Could you check a few things on this model? Use its own coordinates, in mm. Face numbers are marked on the shaded views. A direction names the side the tool comes from. Round coordinates to 2 decimals unless told otherwise and drop trailing zeros. Loops run counter-clockwise (first coordinate to the right, second up) from the corner with the lowest first, then second, coordinate; pieces in that order, holes last. Notation, with made-up numbers: (37, -21.75) -> (71, -21.75) arc R28 ccw to (71, -1.75) -> close; hole circle Ø2 at (89.25, 62.25). An arc over 180 degrees is marked (long way). Write each question's results on one line, items separated by ' | '.
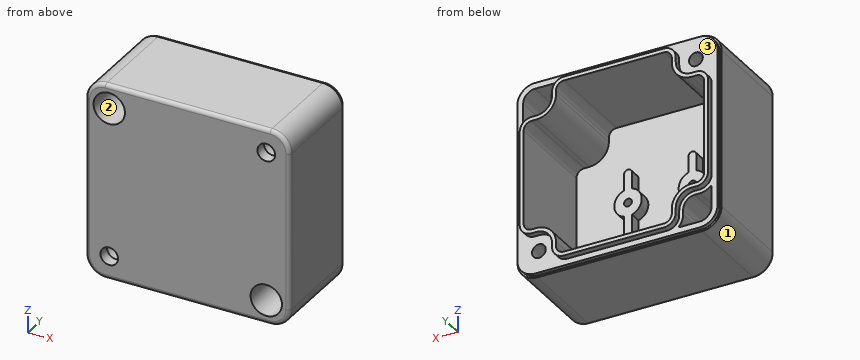
from build123d import *

# Parameters (mm, degrees)
EXTRUDE_1_DEPTH       = 25
CUT_EXTRUDE_START     = 2.5
CUT_EXTRUDE_1_DEPTH   = 22.5
CUT_EXTRUDE_START_2   = 3
CUT_EXTRUDE_3_DEPTH   = 22
EXTRUDE_START         = 25
EXTRUDE_1_2_DEPTH     = 1.6
CUT_EXTRUDE_START_3   = 25
CUT_EXTRUDE_1_2_DEPTH = 1
FILLET_1_R            = 0.2
SKETCH_9_R            = 2.25
CUT_EXTRUDE_4_DEPTH   = 4
SKETCH_10_R           = 4
CUT_EXTRUDE_5_DEPTH   = 17
FILLET_2_R            = 1
SKETCH_11_R           = 1.75
CUT_EXTRUDE_6_DEPTH   = 25
EXTRUDE_2_DEPTH       = 5.5
SKETCH_13_R           = 3.5
EXTRUDE_3_DEPTH       = 5.5
SKETCH_14_R           = 1
CUT_EXTRUDE_7_DEPTH   = 4.5


with BuildPart() as part:
    # Эскиз1 → Extrude 1 (new body)
    with BuildSketch(Plane(origin=(0, 0, 0), x_dir=(1, 0, 0), z_dir=(0, 1, 0))):
        with BuildLine():
            Line((-21, 25), (21, 25))
            ThreePointArc((21, 25), (24.535533906, 23.535533906), (26, 20))
            Line((26, 20), (26, -20))
            ThreePointArc((26, -20), (24.535533906, -23.535533906), (21, -25))
            Line((21, -25), (-21, -25))
            ThreePointArc((-21, -25), (-24.535533906, -23.535533906), (-26, -20))
            Line((-26, -20), (-26, 20))
            ThreePointArc((-26, 20), (-24.535533906, 23.535533906), (-21, 25))
        make_face()
    extrude(amount=EXTRUDE_1_DEPTH)

    # Эскиз2 → Cut-Extrude 1 (cut)
    with BuildSketch(Plane(origin=(0, 0, 0), x_dir=(1, 0, 0), z_dir=(0, 1, 0)).offset(CUT_EXTRUDE_START)):
        with BuildLine():
            Line((-14.75, 20), (-14.75, 18.75))
            ThreePointArc((-14.75, 18.75), (-16.214466094, 15.214466094), (-19.75, 13.75))
            Line((-19.75, 13.75), (-21, 13.75))
            ThreePointArc((-21, 13.75), (-22.414213562, 13.164213562), (-23, 11.75))
            Line((-23, 11.75), (-23, -11.75))
            ThreePointArc((-23, -11.75), (-22.414213562, -13.164213562), (-21, -13.75))
            Line((-21, -13.75), (-19.75, -13.75))
            ThreePointArc((-19.75, -13.75), (-16.214466094, -15.214466094), (-14.75, -18.75))
            Line((-14.75, -18.75), (-14.75, -20))
            ThreePointArc((-14.75, -20), (-14.164213562, -21.414213562), (-12.75, -22))
            Line((-12.75, -22), (12.75, -22))
            ThreePointArc((12.75, -22), (14.164213562, -21.414213562), (14.75, -20))
            Line((14.75, -20), (14.75, -18.955193866))
            ThreePointArc((14.75, -18.955193866), (16.214466094, -15.41965996), (19.75, -13.955193866))
            Line((19.75, -13.955193866), (21, -13.955193866))
            ThreePointArc((21, -13.955193866), (22.414213562, -13.369407428), (23, -11.955193866))
            Line((23, -11.955193866), (23, 11.955193866))
            ThreePointArc((23, 11.955193866), (22.414213562, 13.369407428), (21, 13.955193866))
            Line((21, 13.955193866), (19.75, 13.955193866))
            ThreePointArc((19.75, 13.955193866), (16.214466094, 15.41965996), (14.75, 18.955193866))
            Line((14.75, 18.955193866), (14.75, 20))
            ThreePointArc((14.75, 20), (14.164213562, 21.414213562), (12.75, 22))
            Line((12.75, 22), (-12.75, 22))
            ThreePointArc((-12.75, 22), (-14.164213562, 21.414213562), (-14.75, 20))
        make_face()
    extrude(amount=CUT_EXTRUDE_1_DEPTH, mode=Mode.SUBTRACT)

    # Эскиз8 → Вырез-Вытянуть3 (cut)
    with BuildSketch(Plane(origin=(0, 0, 0), x_dir=(1, 0, 0), z_dir=(0, 1, 0)).offset(CUT_EXTRUDE_START_2)):
        with BuildLine():
            Line((-24, 20), (-24, 14.395751311))
            ThreePointArc((-24, 14.395751311), (-22.645751311, 15.395751311), (-21, 15.75))
            Line((-21, 15.75), (-19.75, 15.75))
            ThreePointArc((-19.75, 15.75), (-17.628679656, 16.628679656), (-16.75, 18.75))
            Line((-16.75, 18.75), (-16.75, 20))
            ThreePointArc((-16.75, 20), (-16.395751311, 21.645751311), (-15.395751311, 23))
            Line((-15.395751311, 23), (-21, 23))
            ThreePointArc((-21, 23), (-23.121320344, 22.121320344), (-24, 20))
        make_face()
        with BuildLine():
            Line((19.75, -15.955193866), (21, -15.955193866))
            ThreePointArc((21, -15.955193866), (22.645751311, -15.600945177), (24, -14.600945177))
            Line((24, -14.600945177), (24, -20))
            ThreePointArc((24, -20), (23.121320344, -22.121320344), (21, -23))
            Line((21, -23), (15.395751311, -23))
            ThreePointArc((15.395751311, -23), (16.395751311, -21.645751311), (16.75, -20))
            Line((16.75, -20), (16.75, -18.955193866))
            ThreePointArc((16.75, -18.955193866), (17.628679656, -16.833873522), (19.75, -15.955193866))
        make_face()
    extrude(amount=CUT_EXTRUDE_3_DEPTH, mode=Mode.SUBTRACT)

    # Эскиз2<2> → Extrude 1 2 (add)
    with BuildSketch(Plane(origin=(0, 0, 0), x_dir=(1, 0, 0), z_dir=(0, 1, 0)).offset(EXTRUDE_START)):
        with BuildLine():
            Line((-19.75, 14.75), (-21, 14.75))
            ThreePointArc((-21, 14.75), (-23.121320344, 13.871320344), (-24, 11.75))
            Line((-24, 11.75), (-24, -11.75))
            ThreePointArc((-24, -11.75), (-23.121320344, -13.871320344), (-21, -14.75))
            Line((-21, -14.75), (-19.75, -14.75))
            ThreePointArc((-19.75, -14.75), (-16.921572875, -15.921572875), (-15.75, -18.75))
            Line((-15.75, -18.75), (-15.75, -20))
            ThreePointArc((-15.75, -20), (-14.871320344, -22.121320344), (-12.75, -23))
            Line((-12.75, -23), (12.75, -23))
            ThreePointArc((12.75, -23), (14.871320344, -22.121320344), (15.75, -20))
            Line((15.75, -20), (15.75, -18.955193866))
            ThreePointArc((15.75, -18.955193866), (16.921572875, -16.126766741), (19.75, -14.955193866))
            Line((19.75, -14.955193866), (21, -14.955193866))
            ThreePointArc((21, -14.955193866), (23.121320344, -14.076514209), (24, -11.955193866))
            Line((24, -11.955193866), (24, 11.955193866))
            ThreePointArc((24, 11.955193866), (23.121320344, 14.076514209), (21, 14.955193866))
            Line((21, 14.955193866), (19.75, 14.955193866))
            ThreePointArc((19.75, 14.955193866), (16.921572875, 16.126766741), (15.75, 18.955193866))
            Line((15.75, 18.955193866), (15.75, 20))
            ThreePointArc((15.75, 20), (14.871320344, 22.121320344), (12.75, 23))
            Line((12.75, 23), (-12.75, 23))
            ThreePointArc((-12.75, 23), (-14.871320344, 22.121320344), (-15.75, 20))
            Line((-15.75, 20), (-15.75, 18.75))
            ThreePointArc((-15.75, 18.75), (-16.921572875, 15.921572875), (-19.75, 14.75))
        make_face()
        with BuildLine():
            Line((-19.75, 13.75), (-21, 13.75))
            ThreePointArc((-21, 13.75), (-22.414213562, 13.164213562), (-23, 11.75))
            Line((-23, 11.75), (-23, -11.75))
            ThreePointArc((-23, -11.75), (-22.414213562, -13.164213562), (-21, -13.75))
            Line((-21, -13.75), (-19.75, -13.75))
            ThreePointArc((-19.75, -13.75), (-16.214466094, -15.214466094), (-14.75, -18.75))
            Line((-14.75, -18.75), (-14.75, -20))
            ThreePointArc((-14.75, -20), (-14.164213562, -21.414213562), (-12.75, -22))
            Line((-12.75, -22), (12.75, -22))
            ThreePointArc((12.75, -22), (14.164213562, -21.414213562), (14.75, -20))
            Line((14.75, -20), (14.75, -18.955193866))
            ThreePointArc((14.75, -18.955193866), (16.214466094, -15.41965996), (19.75, -13.955193866))
            Line((19.75, -13.955193866), (21, -13.955193866))
            ThreePointArc((21, -13.955193866), (22.414213562, -13.369407428), (23, -11.955193866))
            Line((23, -11.955193866), (23, 11.955193866))
            ThreePointArc((23, 11.955193866), (22.414213562, 13.369407428), (21, 13.955193866))
            Line((21, 13.955193866), (19.75, 13.955193866))
            ThreePointArc((19.75, 13.955193866), (16.214466094, 15.41965996), (14.75, 18.955193866))
            Line((14.75, 18.955193866), (14.75, 20))
            ThreePointArc((14.75, 20), (14.164213562, 21.414213562), (12.75, 22))
            Line((12.75, 22), (-12.75, 22))
            ThreePointArc((-12.75, 22), (-14.164213562, 21.414213562), (-14.75, 20))
            Line((-14.75, 20), (-14.75, 18.75))
            ThreePointArc((-14.75, 18.75), (-16.214466094, 15.214466094), (-19.75, 13.75))
        make_face(mode=Mode.SUBTRACT)
    extrude(amount=EXTRUDE_1_2_DEPTH)

    # Эскиз4 → Cut-Extrude 1 2 (cut)
    with BuildSketch(Plane(origin=(0, 0, 0), x_dir=(1, 0, 0), z_dir=(0, 1, 0)).offset(CUT_EXTRUDE_START_3)):
        with BuildLine():
            Line((-26.5, 20), (-26.5, -20))
            ThreePointArc((-26.5, -20), (-24.889087297, -23.889087297), (-21, -25.5))
            Line((-21, -25.5), (21, -25.5))
            ThreePointArc((21, -25.5), (24.889087297, -23.889087297), (26.5, -20))
            Line((26.5, -20), (26.5, 20))
            ThreePointArc((26.5, 20), (24.889087297, 23.889087297), (21, 25.5))
            Line((21, 25.5), (-21, 25.5))
            ThreePointArc((-21, 25.5), (-24.889087297, 23.889087297), (-26.5, 20))
        make_face()
        with BuildLine():
            Line((-25.5, 20), (-25.5, -20))
            ThreePointArc((-25.5, -20), (-24.181980515, -23.181980515), (-21, -24.5))
            Line((-21, -24.5), (21, -24.5))
            ThreePointArc((21, -24.5), (24.181980515, -23.181980515), (25.5, -20))
            Line((25.5, -20), (25.5, 20))
            ThreePointArc((25.5, 20), (24.181980515, 23.181980515), (21, 24.5))
            Line((21, 24.5), (-21, 24.5))
            ThreePointArc((-21, 24.5), (-24.181980515, 23.181980515), (-25.5, 20))
        make_face(mode=Mode.SUBTRACT)
    extrude(amount=-CUT_EXTRUDE_1_2_DEPTH, mode=Mode.SUBTRACT)

    # Скругление1
    fillet_1_edges = [part.edges().sort_by_distance(p)[0] for p in [
        (15.395751311, 14, 23),
        (24, 14, 14.600945177),
        (-15.395751311, 14, -23),
        (-24, 14, -14.395751311),
    ]]
    fillet(fillet_1_edges, radius=FILLET_1_R)

    # Эскиз9 → Вырез-Вытянуть4 (cut)
    with BuildSketch(Plane(origin=(0, 0, 0), x_dir=(1, 0, 0), z_dir=(0, 1, 0))):
        with Locations(Location((-20, 19, 0), (0, 0, 270))):
            Circle(SKETCH_9_R)
        with Locations(Location((20, -19, 0), (0, 0, 270))):
            Circle(SKETCH_9_R)
    extrude(amount=CUT_EXTRUDE_4_DEPTH, mode=Mode.SUBTRACT)

    # Эскиз10 → Вырез-Вытянуть5 (cut)
    with BuildSketch(Plane(origin=(0, 0, 0), x_dir=(1, 0, 0), z_dir=(0, 1, 0))):
        with Locations(Location((20, 19, 0), (0, 0, 270))):
            Circle(SKETCH_10_R)
        with Locations(Location((-20, -19, 0), (0, 0, 270))):
            Circle(SKETCH_10_R)
    extrude(amount=CUT_EXTRUDE_5_DEPTH, mode=Mode.SUBTRACT)

    # Скругление2
    fillet_2_edges = [part.edges().sort_by_distance(p)[0] for p in [
        (0, 0, -25),
        (24.535533906, 0, -23.535533906),
        (26, 0, 0),
        (24.535533906, 0, 23.535533906),
        (0, 0, 25),
        (-24.535533906, 0, 23.535533906),
        (-26, 0, 0),
        (-24.535533906, 0, -23.535533906),
    ]]
    fillet(fillet_2_edges, radius=FILLET_2_R)

    # Эскиз11 → Вырез-Вытянуть6 (cut)
    with BuildSketch(Plane(origin=(0, 0, 0), x_dir=(1, 0, 0), z_dir=(0, 1, 0))):
        with Locations(Location((-20, -19, 0), (0, 0, 90))):
            Circle(SKETCH_11_R)
        with Locations(Location((20, 19, 0), (0, 0, 90))):
            Circle(SKETCH_11_R)
    extrude(amount=CUT_EXTRUDE_6_DEPTH, mode=Mode.SUBTRACT)

    # Эскиз12 → Бобышка-Вытянуть2 (add)
    with BuildSketch(Plane(origin=(0, 0, 0), x_dir=(1, 0, 0), z_dir=(0, 1, 0))):
        with BuildLine():
            Line((-7.2, 7.5), (-7.2, -7.5))
            ThreePointArc((-7.2, -7.5), (-8.2, -8.5), (-9.2, -7.5))
            Line((-9.2, -7.5), (-9.2, 7.5))
            ThreePointArc((-9.2, 7.5), (-8.2, 8.5), (-7.2, 7.5))
        make_face()
    extrude_2 = extrude(amount=EXTRUDE_2_DEPTH)

    # Эскиз13 → Бобышка-Вытянуть3 (add)
    with BuildSketch(Plane(origin=(0, 0, 0), x_dir=(1, 0, 0), z_dir=(0, 1, 0))):
        with Locations((-8.2, 0)):
            Circle(SKETCH_13_R)
    extrude_3 = extrude(amount=EXTRUDE_3_DEPTH)

    # Эскиз14 → Вырез-Вытянуть7 (cut)
    with BuildSketch(Plane(origin=(0, 5.5, 0), x_dir=(1, 0, 0), z_dir=(0, 1, 0))):
        with Locations(Location((-8.2, 0, 0), (0, 0, 270))):
            Circle(SKETCH_14_R)
    cut_extrude_7 = extrude(amount=-CUT_EXTRUDE_7_DEPTH, mode=Mode.SUBTRACT)

    # Зеркальное отражение1: Бобышка-Вытянуть2, Бобышка-Вытянуть3, Вырез-Вытянуть7 across plane
    add(extrude_2.mirror(Plane(origin=(0, 0, 0), x_dir=(0, 0, 1), z_dir=(1, 0, 0))))
    add(extrude_3.mirror(Plane(origin=(0, 0, 0), x_dir=(0, 0, 1), z_dir=(1, 0, 0))))
    add(cut_extrude_7.mirror(Plane(origin=(0, 0, 0), x_dir=(0, 0, 1), z_dir=(1, 0, 0))), mode=Mode.SUBTRACT)


solid = part.part
1) I'm going to push flat-ended pins straight in: pin 1 (0.6 mm diameter, centred on y = 25.5, z = -19, fed in from -X); pin 2 (4 mm diameter, centred on x = 18, z = 19.5, fed in from +Y); pin 3 (0.5 mm diameter, centred on y = 25.5, z = -2, fed in from +X). Where does each tip first touch, or does it pass through?
Model answer:
pin 1: stops at x = -15.75 | pin 2: stops at y = 25 | pin 3: stops at x = 24
2) For the marked faces 1, 2 and 3, which set-ups out of +Z, -Z, +X, -X, +Y, -Y let a thin tool reach every point of the face, with its end or its side?
Model answer:
face 1: -Z, -X, +Y, -Y | face 2: -Y | face 3: +Y
3) I want a section at B-B, the plane x = 19. Give the number of separate pieces and of enclosed holes in the cut face, plus the area to 3 significant figures.
Model answer:
separate pieces: 3 | enclosed holes: 0 | area: 302 mm2
4) I need wall thicknesses on line 1 (X direction, y = 1, z = 19); line 2 (Z direction, x = 20, y = 21.25); line 3 (X direction, y = 17.25, z = 19). Which ranges of each line are inside material? Lowest first, please.
Model answer:
line 1: x = -26 to -24, -16 to 17.75, 22.25 to 26 | line 2: z = -25 to -20.75, -17.25 to -13.96, 13.96 to 15.96, 23 to 25 | line 3: x = -26 to -21.75, -18.25 to -14.75, 14.75 to 16.75, 24 to 26
5) I want a section at C-C, the plane z = 5. Write out the boundary of the cut face in (x, y), plus the area to 3 significant figures.
Model answer:
outline: (-26, 1) arc R1 ccw to (-25, 0) -> (25, 0) arc R1 ccw to (26, 1) -> (26, 24) -> (25.5, 24) -> (25.5, 25) -> (24, 25) -> (24, 26.6) -> (23, 26.6) -> (23, 2.5) -> (9.2, 2.5) -> (9.2, 5.5) -> (7.2, 5.5) -> (7.2, 2.5) -> (-7.2, 2.5) -> (-7.2, 5.5) -> (-9.2, 5.5) -> (-9.2, 2.5) -> (-23, 2.5) -> (-23, 26.6) -> (-24, 26.6) -> (-24, 25) -> (-25.5, 25) -> (-25.5, 24) -> (-26, 24) -> close | area: 279 mm2
6) I want a section at A-A, the plane x = 8.2. Write out the boundary of the cut face in (y, z).
Model answer:
outline: (0, -24) arc R1 ccw to (1, -25) -> (24, -25) -> (24, -24.5) -> (25, -24.5) -> (25, -23) -> (26.6, -23) -> (26.6, -22) -> (2.5, -22) -> (2.5, -8.5) -> (5.5, -8.5) -> (5.5, -1) -> (1, -1) -> (1, 1) -> (5.5, 1) -> (5.5, 8.5) -> (2.5, 8.5) -> (2.5, 22) -> (26.6, 22) -> (26.6, 23) -> (25, 23) -> (25, 24.5) -> (24, 24.5) -> (24, 25) -> (1, 25) arc R1 ccw to (0, 24) -> close
